Can you work these out from the model? Positions are in its coordinate system, mm. A direction names the side the tool comes from. Round coordinates to 2 decimals unless told otherwise and drop trailing zeros. Order: outer loops, then holes, each group sorted by start corner. A loop starts at its lowest first (then second) coordinate and runs counter-clockwise, first axis right, second up.
from build123d import *

# Parameters (mm, degrees)
EXTRUDE_1_DEPTH     = 21
SKETCH_4_R          = 1.5
CUT_EXTRUDE_1_DEPTH = 6
SKETCH_5_R          = 1.5
EXTRUDE_2_DEPTH     = 6


with BuildPart() as part:
    # 草图3 → 凸台-拉伸1 (new body)
    with BuildSketch(Plane.XY):
        Polygon((1.6, 2.771281292), (-1.6, 2.771281292), (-3.2, 0), (-1.6, -2.771281292), (1.6, -2.771281292), (3.2, 0), align=None)
    extrude(amount=EXTRUDE_1_DEPTH)

    # 草图4 → 切除-拉伸1 (cut)
    with BuildSketch(Plane(origin=(0, 0, 0), x_dir=(-1, 0, 0), z_dir=(0, 0, -1))):
        Circle(SKETCH_4_R)
    extrude(amount=-CUT_EXTRUDE_1_DEPTH, mode=Mode.SUBTRACT)

    # 草图5 → 凸台-拉伸2 (add)
    with BuildSketch(Plane.XY.offset(21)):
        with Locations(Location((0, 0, 0), (0, 0, 180))):
            Circle(SKETCH_5_R)
    extrude(amount=EXTRUDE_2_DEPTH)


solid = part.part
(1) I want a section at A-A, the plane z = 5. List the corners of the cut face in (x, y) for me.
(2) On a 3-axis mill with a long thin cutter (end or side, diameter ignored), from which of +Z, -Z, +X, -X, +Y, -Y can I reach the whole of each face in a straight line? I mean faces 4 (the face through (0, 2.771, 10)), 5 (the face through (1.5, 0.07, 2.96)), 6 (the face through (-1.43, -0.45, 23.96)). Say none if no direction works.
(3) I want a section at B-B, the plane y = -0.55. List the corners of the cut face in (x, z) for me.
(4) Please list where these lines run through material, in increasing order: probe 1 along Y at (x, z) = (0, 3); probe 2 along Z at (x, y) = (-2.5, 1); probe 3 along Z at (x, y) = (-0.75, 0).
(5) I want a section at C-C, the plane x = -1. List the corners of the cut face in (y, z) for me, plus the area to 3 significant figures.
(6) I want a section at D-D, the plane z = 8.5. List the corners of the cut face in (x, y) for me, plus the area to 3 significant figures.
(7) If we mould it in two halves opening along X, with no side actions, what happens to faces 1 (the face through (2.389, -1.405, 10.353)), 2 (the face through (0, 0, 6)), 3 (the face through (0, -2.771, 10))? For each: pulls with the +X half, pulls with the -X half, needs draft (parallel to the pull), parting line crosses it, or undercut.
Ans:
1. outline: (-3.2, 0) - (-1.6, -2.77) - (1.6, -2.77) - (3.2, 0) - (1.6, 2.77) - (-1.6, 2.77) - close; hole circle Ø3 at (0, 0)
2. face 4: +Z, -Z, +X, -X, +Y
2. face 5: -Z
2. face 6: +Z
3. outline: (-2.88, 0) - (-1.4, 0) - (-1.4, 6) - (1.4, 6) - (1.4, 0) - (2.88, 0) - (2.88, 21) - (1.4, 21) - (1.4, 27) - (-1.4, 27) - (-1.4, 21) - (-2.88, 21) - close
4. probe 1: y = -2.77 to -1.5, 1.5 to 2.77
4. probe 2: z = 0 to 21
4. probe 3: z = 6 to 27
5. outline: (-2.77, 0) - (-1.12, 0) - (-1.12, 6) - (1.12, 6) - (1.12, 0) - (2.77, 0) - (2.77, 21) - (1.12, 21) - (1.12, 27) - (-1.12, 27) - (-1.12, 21) - (-2.77, 21) - close
5. area: 116 mm2
6. outline: (-3.2, 0) - (-1.6, -2.77) - (1.6, -2.77) - (3.2, 0) - (1.6, 2.77) - (-1.6, 2.77) - close
6. area: 26.6 mm2
7. face 1: pulls with the +X half
7. face 2: undercut
7. face 3: needs draft
